Part model, mm, in its own coordinate system. Face numbers are marked on the shaded views. Give positions to 0.01 mm unless a question says otherwise; leave off trailing zeros. Write each loop counter-clockwise with the first axis right and the second up, starting at its lowest first coordinate (ties: lowest second). Pieces come first, ordered by that corner, then holes. Notation, with made-up numbers: M 74,0.5 L 78,0.5 A12 cw 78,12.5 Z; hole C 0,42 d4. An arc over 180 degrees is marked long. Write item = value, one per line. Start each with the question number.
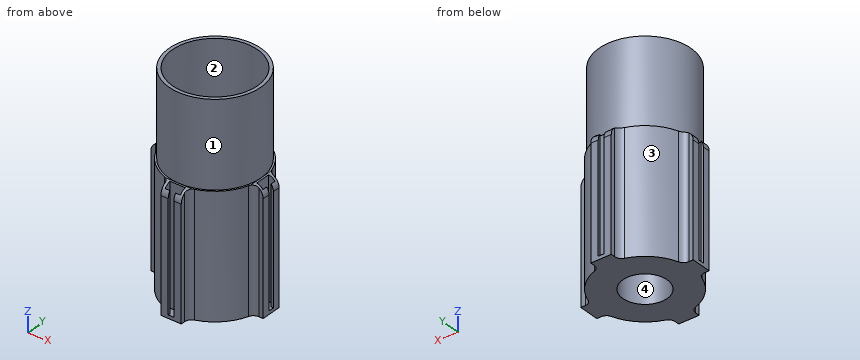
from build123d import *

# Parameters (mm, degrees)
CROQUIS1_R                 = 14
SALIENTE_EXTRUIR1_DEPTH    = 36
CROQUIS2_R                 = 6.55
CORTAR_EXTRUIR1_DEPTH      = 33
CROQUIS3_R                 = 4.5
CORTAR_EXTRUIR2_DEPTH      = 1
VACIADO3_START             = -36
VACIADO3_OUTLINE_R         = 14
VACIADO3_OUTLINE_R_2       = 7.55
VACIADO3_DEPTH             = 36
VACIADO3_2_OUTLINE_R       = 7.55
VACIADO3_2_DEPTH           = 1
VACIADO3_START_2           = -35
VACIADO3_3_OUTLINE_R       = 7.55
VACIADO3_3_OUTLINE_R_2     = 5.5
VACIADO3_3_DEPTH           = 1
CROQUIS4_R                 = 14
CROQUIS4_R_2               = 13
EXTRUIR_L_MINA1_DEPTH      = 36
CROQUIS11_R                = 13
SALIENTE_EXTRUIR2_DEPTH    = 2
CORTAR_EXTRUIR8_REACH      = 41.345
CROQUIS20_R                = 4.5
SALIENTE_EXTRUIR6_START    = -0.325206
SALIENTE_EXTRUIR6_DEPTH    = 2.825206
CORTAR_EXTRUIR9_DEPTH      = 35
CROQUIS31_R                = 13
CROQUIS31_R_2              = 7
EXTRUIR_L_MINA2_DEPTH      = 0.5
CROQUIS33_R                = 13.5
CROQUIS33_R_2              = 12.5
EXTRUIR_L_MINA3_DEPTH      = 25
REDONDEO2_R                = 2
REDONDEO6_R                = 3
MATRIZC1_COUNT             = 4
REDONDEO2_OF_MATRIZC1_R    = 2
REDONDEO6_OF_MATRIZC1_R    = 3
CHAFL_N2_SIZE              = 2.300736814
CHAFL_N2_SIZE2             = 2
CHAFL_N4_SIZE              = 6
S_LIDO_MOVER_COPIAR2_ANGLE = 180
CROQUIS35_R                = 2.5
CORTAR_EXTRUIR11_DEPTH     = 0.585651992
MATRIZC2_COUNT             = 10
CROQUIS38_R                = 6.75
CROQUIS38_R_2              = 6.5
EXTRUIR_L_MINA4_DEPTH      = 15


# Read off the part's stored shape, not the designer's step: Vaciado3
# Some blends are built 0.0001 mm under size
with BuildPart() as part:
    # Croquis1 → Saliente-Extruir1 (new body)
    with BuildSketch(Plane.XY):
        Circle(CROQUIS1_R)
    extrude(amount=-SALIENTE_EXTRUIR1_DEPTH)

    # Croquis2 → Cortar-Extruir1 (cut)
    with BuildSketch(Plane.XY):
        Circle(CROQUIS2_R)
    extrude(amount=-CORTAR_EXTRUIR1_DEPTH, mode=Mode.SUBTRACT)

    # Croquis3 → Cortar-Extruir2 (cut)
    with BuildSketch(Plane.XY.offset(-33)):
        Circle(CROQUIS3_R)
    extrude(amount=-CORTAR_EXTRUIR2_DEPTH, mode=Mode.SUBTRACT)

    # Vaciado3 outline → Vaciado3 (cut)
    with BuildSketch(Plane.XY.offset(VACIADO3_START)):
        Circle(VACIADO3_OUTLINE_R)
        Circle(VACIADO3_OUTLINE_R_2, mode=Mode.SUBTRACT)
    extrude(amount=VACIADO3_DEPTH, mode=Mode.SUBTRACT)

    # Vaciado3 2 outline → Vaciado3 2 (cut)
    with BuildSketch(Plane.XY.offset(VACIADO3_START)):
        Circle(VACIADO3_2_OUTLINE_R)
    extrude(amount=VACIADO3_2_DEPTH, mode=Mode.SUBTRACT)

    # Vaciado3 3 outline → Vaciado3 3 (cut)
    with BuildSketch(Plane.XY.offset(VACIADO3_START_2)):
        Circle(VACIADO3_3_OUTLINE_R)
        Circle(VACIADO3_3_OUTLINE_R_2, mode=Mode.SUBTRACT)
    extrude(amount=VACIADO3_3_DEPTH, mode=Mode.SUBTRACT)



with BuildPart() as body_2:
    # Croquis4 → Extruir-Lámina1 (new body)
    with BuildSketch(Plane.XY):
        Circle(CROQUIS4_R)
        Circle(CROQUIS4_R_2, mode=Mode.SUBTRACT)
    extrude(amount=-EXTRUIR_L_MINA1_DEPTH)


with BuildPart() as part_1:
    add(part.part)

    add(body_2.part)  # Saliente-Extruir2 merges body 2
    # Croquis11 → Saliente-Extruir2 (add)
    with BuildSketch(Plane.XY.offset(-34)):
        Circle(CROQUIS11_R)
    extrude(amount=-SALIENTE_EXTRUIR2_DEPTH)

    # Croquis20 → Cortar-Extruir8 (cut, up to next)
    with BuildSketch(Plane.XY.offset(-34), mode=Mode.PRIVATE) as cortar_extruir8_sk1:
        Circle(CROQUIS20_R)
    cortar_extruir8_tool1 = extrude(cortar_extruir8_sk1.sketch, amount=-CORTAR_EXTRUIR8_REACH, mode=Mode.PRIVATE) & part_1.part
    add(cortar_extruir8_tool1.solids().sort_by_distance((0, 0, -34))[0], mode=Mode.SUBTRACT)

    # Croquis21 → Saliente-Extruir6 (add)
    with BuildSketch(Plane(origin=(0, 14, 0), x_dir=(1, 0, 0), z_dir=(0, 1, 0)).offset(SALIENTE_EXTRUIR6_START)):
        Polygon((0, 0), (-3, 0), (-3, 36), (3, 36), (3, 0), align=None)
    saliente_extruir6 = extrude(amount=SALIENTE_EXTRUIR6_DEPTH)

    # Croquis29 → Cortar-Extruir9 (cut)
    with BuildSketch(Plane(origin=(0, 0, -36), x_dir=(-1, 0, 0), z_dir=(0, 0, -1))):
        Polygon((-2.25, 14), (2.25, 14), (2.25, 15.85), (0.825, 15.85), (0.825, 16.5), (-0.825, 16.5), (-0.825, 15.85), (-2.25, 15.85), align=None)
    cortar_extruir9 = extrude(amount=-CORTAR_EXTRUIR9_DEPTH, mode=Mode.SUBTRACT)

    # Croquis31 → Extruir-Lámina2 (add)
    with BuildSketch(Plane.XY):
        Circle(CROQUIS31_R)
        Circle(CROQUIS31_R_2, mode=Mode.SUBTRACT)
    extrude(amount=-EXTRUIR_L_MINA2_DEPTH)

    # Croquis33 → Extruir-Lámina3 (add)
    with BuildSketch(Plane(origin=(0, 0, -36), x_dir=(-1, 0, 0), z_dir=(0, 0, -1))):
        Circle(CROQUIS33_R)
        Circle(CROQUIS33_R_2, mode=Mode.SUBTRACT)
    extrude(amount=EXTRUIR_L_MINA3_DEPTH)

    # Redondeo2
    redondeo2_edges = [part_1.edges().sort_by_distance(p)[0] for p in [
        (-3, 13.674794, -18),
        (3, 13.674794, -18),
    ]]
    fillet(redondeo2_edges, radius=REDONDEO2_R)

    # Redondeo6
    # the kernel refuses this fillet: 3 mm, written as the material it takes off along each edge
    with BuildSketch(Plane(origin=(-10.5, 16.5, -36), x_dir=(0, 0, 1), z_dir=(1, 0, 0))) as redondeo6_piece_1:
        with BuildLine():
            CenterArc((REDONDEO6_R, REDONDEO6_R), REDONDEO6_R, 180, 90)
            Line((0, REDONDEO6_R), (0, 0))
            Line((0, 0), (REDONDEO6_R, 0))
        make_face()
    extrude(amount=17.175, mode=Mode.SUBTRACT)

    # MatrizC1: Saliente-Extruir6, Cortar-Extruir9 ×4 about axis
    matrizc1_axis = Axis((0, 0, 0), (0, 0, 1))
    add([saliente_extruir6.rotate(matrizc1_axis, i * 360 / MATRIZC1_COUNT) for i in range(1, MATRIZC1_COUNT)])
    add([cortar_extruir9.rotate(matrizc1_axis, i * 360 / MATRIZC1_COUNT) for i in range(1, MATRIZC1_COUNT)], mode=Mode.SUBTRACT)

    # Redondeo2 of MatrizC1
    redondeo2_of_matrizc1_edges = [part_1.edges().sort_by_distance(p)[0] for p in [
        (-13.674794, -3, -18),
        (-13.674794, 3, -18),
        (3, -13.674794, -18),
        (-3, -13.674794, -18),
        (13.674794, 3, -18),
        (13.674794, -3, -18),
    ]]
    fillet(redondeo2_of_matrizc1_edges, radius=REDONDEO2_OF_MATRIZC1_R)

    # Redondeo6 of MatrizC1
    # the kernel refuses this fillet: 3 mm, written as the material it takes off along each edge
    with BuildSketch(Plane(origin=(-16.5, -10.5, -36), x_dir=(0, 0, 1), z_dir=(0, 1, 0)), Plane(origin=(10.5, -16.5, -36), x_dir=(0, 0, 1), z_dir=(-1, 0, 0)), Plane(origin=(16.5, 10.5, -36), x_dir=(0, 0, 1), z_dir=(0, -1, 0))) as redondeo6_of_matrizc1_piece_1:
        with BuildLine():
            CenterArc((REDONDEO6_OF_MATRIZC1_R, REDONDEO6_OF_MATRIZC1_R), REDONDEO6_OF_MATRIZC1_R, 180, 90)
            Line((0, REDONDEO6_OF_MATRIZC1_R), (0, 0))
            Line((0, 0), (REDONDEO6_OF_MATRIZC1_R, 0))
        make_face()
    extrude(amount=17.175, mode=Mode.SUBTRACT)

    # Chaflán2
    chafl_n2_edges = [part_1.edges().sort_by_distance(p)[0] for p in [
        (-4.5, 0, -36),
    ]]
    chafl_n2_side = [part_1.faces().sort_by_distance(p)[0] for p in [
        (-4.5, 0, -34.5),
    ]]
    chamfer(chafl_n2_edges, length=CHAFL_N2_SIZE, length2=CHAFL_N2_SIZE2, reference=chafl_n2_side[0])

    # Chaflán4
    chafl_n4_edges = [part_1.edges().sort_by_distance(p)[0] for p in [
        (12.5, 0, -36),
    ]]
    chamfer(chafl_n4_edges, length=CHAFL_N4_SIZE - 0.0001)  # a hair under: the kernel refuses the full size


with BuildPart() as part_2:
    # Sólido-Mover/Copiar2: moved
    add(part_1.part.rotate(Axis((0, 0, 0), (0, 1, 0)), S_LIDO_MOVER_COPIAR2_ANGLE))

    # Croquis34 → Cortar-Revolución1 (revolve, cut)
    with BuildSketch(Plane(origin=(0, 0, 0), x_dir=(1, 0, 0), z_dir=(0, 1, 0))):
        Polygon((-12.5, -40.763390042), (-12.5, -34.585651992), (-6.995999587, -34.585651992), align=None)
    revolve(axis=Axis((0, 0, -36), (0, 0, 1)), mode=Mode.SUBTRACT)

    # Croquis35 → Cortar-Extruir11 (cut)
    with BuildSketch(Plane(origin=(0, 0, 34), x_dir=(-1, 0, 0), z_dir=(0, 0, -1))):
        with Locations((-10.25, 0)):
            Circle(CROQUIS35_R)
    cortar_extruir11 = extrude(amount=-CORTAR_EXTRUIR11_DEPTH, mode=Mode.SUBTRACT)

    # MatrizC2: Cortar-Extruir11 ×10 about axis
    matrizc2_axis = Axis((0, 0, 0), (0, 0, 1))
    for i in range(1, MATRIZC2_COUNT):
        add(cortar_extruir11.rotate(matrizc2_axis, i * 360 / MATRIZC2_COUNT), mode=Mode.SUBTRACT)

    # Croquis38 → Extruir-Lámina4 (add)
    with BuildSketch(Plane(origin=(0, 0, 0), x_dir=(-1, 0, 0), z_dir=(0, 0, -1))):
        Circle(CROQUIS38_R)
        Circle(CROQUIS38_R_2, mode=Mode.SUBTRACT)
    extrude(amount=-EXTRUIR_L_MINA4_DEPTH)


solid = part_2.part
Q1. Two-plate mould, pull along X, no slides. Class the marked faces 1, 2, 3 and 4: +X half, -X half, draft (parallel to the pull), parting line (faces both ways), or undercut.
Q2. Slice it at A-A (z = 31.5). Give the number of separate pieces and of enclosed holes in the cut face, and give its area (3 significant figures).
Q3. Drop flat-ended pins along their axis: P1, Ø2, axis at x = -15, z = 16, coming from the +Y side; P2, Ø5, axis at x = -7.5, z = 41, coming from the -Y side; P3, Ø4, axis at x = -1.5, z = 50, coming from the -Y side. Give the stop position or say it passes through.
Q4. Slice it at B-B (z = 57.5). Give the cut face in (x, y), and give its area (3 significant figures).
Q5. Slice it at D-D (z = 38.5). Give the cut face in (x, y).
Q6. Probe line 1 along Y through (x, z) = (0, 26); line 2 along Z through (x, y) = (8, 10); line 3 along Z through (x, y) = (5, 6.5). List the from-to ranges inside material, lowest first.
Working result:
q1.face_1 = parting line
q1.face_2 = undercut
q1.face_3 = -X half
q1.face_4 = undercut
q2.separate_pieces = 2
q2.enclosed_holes = 2
q2.area = 158 mm2
q3.P1 = 3.4
q3.P2 = -12.54
q3.P3 = -13.5
q4.outline = C 0,0 d27; hole C 0,0 d25
q4.area = 81.7 mm2
q5.outline = C 0,0 d27; C 0,0 d20.97; hole C 0,0 d25; hole C 0,0 d18
q6.line_1 = -14 to -13, -7.55 to -6.55, 6.55 to 7.55, 13 to 14
q6.line_2 = 0 to 0.5, 34 to 61
q6.line_3 = 0 to 0.5, 34 to 34.59, 35.94 to 37.7
